```python
from build123d import *

# Parameters (mm, degrees)
F0_R     = 55
F1_DEPTH = 7.2
F2_R     = 2.25
F5_DEPTH = 7.2
F6_R     = 4.5
F7_DEPTH = 30
F8_R     = 45
F9_DEPTH = 37.201


with BuildPart() as f1:
    # F0 (on Top) → F1 (new body)
    with BuildSketch(Plane.XY):
        Circle(F0_R)
    extrude(amount=F1_DEPTH)

    # F3 (on Front) → F4 (revolve)
    with BuildSketch(Plane.XZ):
        Polygon((0, 37.2), (0, 7.2), (50, 7.2), (50, 10.2), (53.5, 10.2), (53.5, 13.2), (50, 13.2), (50, 16.2), (53.5, 16.2), (53.5, 19.2), (50, 19.2), (50, 22.2), (53.5, 22.2), (53.5, 25.2), (50, 25.2), (50, 28.2), (53.5, 28.2), (53.5, 31.2), (50, 31.2), (50, 34.2), (53.5, 34.2), (53.5, 37.2), align=None)
    revolve(axis=Axis((0, 0, 22.2), (0, 0, -1)))

    # F2 (on face) → F5 (cut, through all)
    with BuildSketch(Plane.XY.offset(7.2)):
        with Locations((-35.75, 35.75)):
            Circle(F2_R)
        with Locations((-35.75, -35.75)):
            Circle(F2_R)
        with Locations((35.75, -35.75)):
            Circle(F2_R)
        with Locations((35.75, 35.75)):
            Circle(F2_R)
    extrude(amount=-F5_DEPTH, mode=Mode.SUBTRACT)

    # F6 (on face) → F7 (cut, through all)
    with BuildSketch(Plane.XY.offset(37.2)):
        with Locations((-35.75, 35.75)):
            Circle(F6_R)
        with Locations((-35.75, -35.75)):
            Circle(F6_R)
        with Locations((35.75, -35.75)):
            Circle(F6_R)
        with Locations((35.75, 35.75)):
            Circle(F6_R)
    extrude(amount=-F7_DEPTH, mode=Mode.SUBTRACT)

    # F8 (on face) → F9 (cut, through all)
    with BuildSketch(Plane.XY.offset(37.2)):
        Circle(F8_R)
    extrude(amount=-F9_DEPTH, mode=Mode.SUBTRACT)


solid = f1.part
```
Input: part model. Units: mm. Frame: model coordinates. A direction names the side the tool comes from. Give positions to 0.01 mm unless a question says otherwise; leave off trailing zeros.
1. Pin query (flat end, axial travel): pin 1 (8 mm diameter, centred on x = -35.75, y = 35.75, fed in from +Z); pin 2 (7.5 mm diameter, centred on x = -44, y = -3, fed in from -Z); pin 3 (8 mm diameter, centred on x = -36.5, z = 27, fed in from -Y); pin 4 (1.5 mm diameter, centred on x = 38, z = 23.5, fed in from -Y). Return the tip coordinate at first contact, or that it passes through.
Derived:
pin 1: stops at z = 7.2
pin 2: stops at z = 0
pin 3: stops at y = -42.36
pin 4: stops at y = -32.4
2. Reachability of faces 1 (the flat face through (50.4, -2.8, 16.2)), 2 (the cylindrical face through (-53.497, -0.539, 17.721)), 3 (the flat face through (-50.4, -2.8, 25.2)), 4 (the flat face through (0.2, -50.4, 10.2)) from +Z, -Z, +X, -X, +Y, -Y: full face, straight path, thin tool, end or side. Return the list, or none.
Derived:
face 1: +X
face 2: +Z, -X
face 3: -X
face 4: -Y
3. Material intervals for L1, parallel to Z at x = 42.5, y = -29.5; L2, parallel to X at y = 35, z = 4; L3, parallel to X at y = -32, z = 22, sorted ascending.
Derived:
L1: z = 0 to 7.2, 10.2 to 13.2, 16.2 to 19.2, 22.2 to 25.2, 28.2 to 31.2, 34.2 to 37.2
L2: x = -42.43 to -37.87, -33.63 to -28.28, 28.28 to 33.63, 37.87 to 42.43
L3: x = -38.42 to -38.24, -33.26 to -31.64, 31.64 to 33.26, 38.24 to 38.42
